CAD build for the part. Positions are in the model's coordinates, mm. Round coordinates to 2 decimals unless told otherwise and drop trailing zeros. Order: outer loops, then holes, each group sorted by start corner. A loop starts at its lowest first (then second) coordinate and runs counter-clockwise, first axis right, second up. Notation, with made-up numbers: (64.5, 40.5) -> (116.5, 40.5) arc R20 ccw to (116.5, 68.5) -> close; hole circle Ø5 at (43, -22). An arc over 180 degrees is marked (long way). Return JSON: item names as keys, results as strings. Group by question number.
Q1. Cut at C-C (x = 36). Write the cut outline in (y, z), then the cut area to 3 significant figures.
Q2. Cut at B-B (z = 0). Write the cut outline in (x, y) (3 decimals).
Q3. Flat gauge pins, fed straight in: pin 1 (5.5 mm diameter, centred on y = -20.55, z = 0, fed in from +X); pin 2 (3 mm diameter, centred on x = 62.5, z = -1, fed in from +Y); pin 3 (12 mm diameter, centred on x = 52.5, y = 11, fed in from +Z); pin 4 (7 mm diameter, centred on y = 0, z = 0, fed in from -X). Where does each tip first touch, or does it go through?
Q4. Probe line 1 along Y through (x, z) = (1.3, 0) (3 decimals); line 2 along X through (y, z) = (-14, -4.5); line 3 along Z through (x, y) = (43, 44). List the from-to ranges inside material, lowest first.
Q5. Cut at A-A (y = 0). Write the cut outline in (x, z) (3 decimals).
Q6. Cut at D-D (z = -42). Write the cut outline in (x, y), then the cut area to 3 significant figures.
from build123d import *

# Parameters (mm, degrees)
ESQUISSE1_R             = 50
BOSS_EXTRU_1_DEPTH      = 5
ESQUISSE2_R             = 3
BOSS_EXTRU_3_DEPTH      = 70
ESQUISSE3_R             = 2.125
ENL_V_MAT_EXTRU_2_DEPTH = 70


with BuildPart() as part:
    # Esquisse1 → Boss.-Extru.1 (new body)
    with BuildSketch(Plane(origin=(0, 0, 0), x_dir=(0, 0, -1), z_dir=(1, 0, 0))):
        Circle(ESQUISSE1_R)
    extrude(amount=BOSS_EXTRU_1_DEPTH)

    # Esquisse2 → Boss.-Extru.3 (add)
    with BuildSketch(Plane(origin=(5, 0, 0), x_dir=(0, 0, -1), z_dir=(1, 0, 0))):
        with Locations((-42, 0)):
            Circle(ESQUISSE2_R)
        with Locations((42, 0)):
            Circle(ESQUISSE2_R)
        with Locations((0, -42)):
            Circle(ESQUISSE2_R)
        with Locations((0, 42)):
            Circle(ESQUISSE2_R)
    extrude(amount=BOSS_EXTRU_3_DEPTH)

    # Esquisse3 → Enlèv. mat.-Extru.2 (cut)
    with BuildSketch(Plane(origin=(5, 0, 0), x_dir=(0, 0, -1), z_dir=(1, 0, 0))):
        Circle(ESQUISSE3_R)
        with Locations((0, -20.547843558)):
            Circle(ESQUISSE3_R)
    extrude(amount=-ENL_V_MAT_EXTRU_2_DEPTH, mode=Mode.SUBTRACT)


solid = part.part
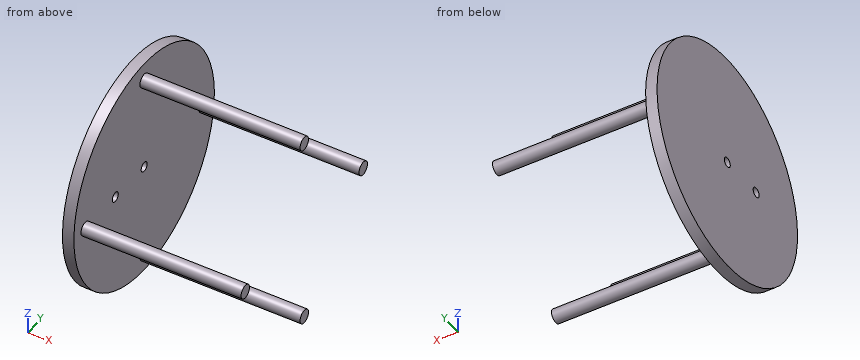
Solution:
{
 "1": {"outline": "circle Ø6 at (-42, 0); circle Ø6 at (0, -42); circle Ø6 at (0, 42); circle Ø6 at (42, 0)", "area": "113 mm²"},
 "2": {"outline": "(0, -50) -> (5, -50) -> (5, -45) -> (75, -45) -> (75, -39) -> (5, -39) -> (5, -22.673) -> (0, -22.673) -> close; (0, -18.423) -> (5, -18.423) -> (5, -2.125) -> (0, -2.125) -> close; (0, 2.125) -> (5, 2.125) -> (5, 39) -> (75, 39) -> (75, 45) -> (5, 45) -> (5, 50) -> (0, 50) -> close"},
 "3": {"pin 1": "stops at x = 5", "pin 2": "stops at y = 45", "pin 3": "passes through", "pin 4": "stops at x = 0"},
 "4": {"line 1": "y = -50 to -22.673, -18.423 to -2.125, 2.125 to 50", "line 2": "x = 0 to 5", "line 3": "z = -2.24 to 2.24"},
 "5": {"outline": "(0, -50) -> (5, -50) -> (5, -45) -> (75, -45) -> (75, -39) -> (5, -39) -> (5, -2.125) -> (0, -2.125) -> close; (0, 2.125) -> (5, 2.125) -> (5, 39) -> (75, 39) -> (75, 45) -> (5, 45) -> (5, 50) -> (0, 50) -> close"},
 "6": {"outline": "(0, -27.13) -> (5, -27.13) -> (5, -3) -> (75, -3) -> (75, 3) -> (5, 3) -> (5, 27.13) -> (0, 27.13) -> close", "area": "691 mm²"}
}
